from build123d import *

# Parameters (mm, degrees)
SKETCH3_W           = 90
SKETCH3_H           = 50
BOSS_EXTRUDE1_DEPTH = 10
BOSS_EXTRUDE2_DEPTH = 24
SKETCH5_R           = 20
BOSS_EXTRUDE3_DEPTH = 26
SKETCH6_W           = 20
SKETCH6_H           = 27.110350909
CUT_EXTRUDE1_DEPTH  = 15
SKETCH7_W           = 26.369202788
SKETCH7_H           = 10.718734527
CUT_EXTRUDE2_DEPTH  = 35
SKETCH9_W           = 20
SKETCH9_H           = 12
CUT_EXTRUDE3_DEPTH  = 114.798066767


with BuildPart() as part:
    # Sketch3 → Boss-Extrude1 (new body)
    with BuildSketch(Plane.XY):
        Rectangle(SKETCH3_W, SKETCH3_H)
    extrude(amount=BOSS_EXTRUDE1_DEPTH)

    # Sketch4 → Boss-Extrude2 (add)
    with BuildSketch(Plane.XZ.offset(25)):
        Polygon((45, 10), (-45, 10), (-25, 60), (25, 60), align=None)
    extrude(amount=-BOSS_EXTRUDE2_DEPTH)

    # Sketch5 → Boss-Extrude3 (add)
    with BuildSketch(Plane(origin=(0, -1, 0), x_dir=(1, 0, 0), z_dir=(0, 1, 0))):
        with Locations(Location((0, -45, 0), (0, 0, 311.409622109))):
            Circle(SKETCH5_R)
    extrude(amount=BOSS_EXTRUDE3_DEPTH)

    # Sketch6 → Cut-Extrude1 (cut)
    with BuildSketch(Plane(origin=(0, 25, 0), x_dir=(1, 0, 0), z_dir=(0, 1, 0))):
        with Locations((0, -31.444824546)):
            Rectangle(SKETCH6_W, SKETCH6_H)
    extrude(amount=-CUT_EXTRUDE1_DEPTH, mode=Mode.SUBTRACT)

    # Sketch7 → Cut-Extrude2 (cut)
    with BuildSketch(Plane.XZ.offset(25)):
        with Locations((-0.044155161, 65.359367264)):
            Rectangle(SKETCH7_W, SKETCH7_H)
    extrude(amount=-CUT_EXTRUDE2_DEPTH, mode=Mode.SUBTRACT)

    # Sketch9 → Cut-Extrude3 (cut, through all)
    with BuildSketch(Plane(origin=(45, 0, 0), x_dir=(0, 0, -1), z_dir=(1, 0, 0))):
        with Locations((-35, -13)):
            Rectangle(SKETCH9_W, SKETCH9_H)
    extrude(amount=-CUT_EXTRUDE3_DEPTH, mode=Mode.SUBTRACT)


solid = part.part
Read the model definition and answer for the solid it produces. Units are mm, in the model's axes. A direction names the side the tool comes from. Round coordinates to 2 decimals unless told otherwise and drop trailing zeros. Write each loop counter-clockwise with the first axis right and the second up, starting at its lowest first coordinate (ties: lowest second). Pieces come first, ordered by that corner, then holes. Notation, with made-up numbers: (-2.5, 24.5) - (38.5, 24.5) arc R28 ccw to (38.5, 52.5) - close; hole circle Ø4 at (-7, -3.5). An arc over 180 degrees is marked (long way). One line per question, with ' | ' between items. Start each with the question number.
1. Section C-C (z = 31.5) is taken. Determine the outline of the cut face in (x, y), and give its area (3 significant figures).
2. Section A-A (y = -12) is taken. Determine the outline of the cut face in (x, z).
3. Section B-B (x = 30) is taken. Determine the outline of the cut face in (y, z), and give its area (3 significant figures).
4. For a pull along Y with two mould halves and no side action, classify faces 6 (the face through (1, -7, 35)), 7 (the face through (0, -12, 60)), 8 (the face through (0, 10, 35)) as +Y half, -Y half, draft (parallel to the pull), parting line (faces both ways), or undercut.
5. Find the intervals of material crossed by probe 1 along Z at (x, y) = (24, -18); probe 2 along Y at (x, z) = (11.5, 37); probe 3 along Y at (x, z) = (27, 33.5), in increasing order. Write a range as [from, to].
6. Each of these flat-tipped pins is pushed along its axis until it touches: pin 1 (16.5 mm diameter, centred on y = 15.5, z = 36.5, fed in from +X); pin 2 (6 mm diameter, centred on x = 0, z = 39.5, fed in from +Y); pin 3 (1.5 mm diameter, centred on y = 19, z = 54.5, fed in from +X). Where does it stop, or does it pass through?
7. Section D-D (y = 7) is taken. Determine the outline of the cut face in (x, z), and give its area (3 significant figures).
8. For faces 1 (the face through (-1, 12, 10)), 2 (the face through (0, -13, 45)), 3 (the face through (1, -25, 30)), 4 (the face through (-45, 0, 5)), 5 (the face through (0, 18, 45)), determine the directions among +Z, -Z, +X, -X, +Y, -Y from which every point of the face is accessible in a straight line to the end or side of a thin tool.
Filled in:
1) outline: (-36.4, -25) - (36.4, -25) - (36.4, -19) - (-36.4, -19) - close; (-36.4, -7) - (36.4, -7) - (36.4, -1) - (14.76, -1) - (14.76, 25) - (10, 25) - (10, 10) - (-10, 10) - (-10, 25) - (-14.76, 25) - (-14.76, -1) - (-36.4, -1) - close | area: 1,340 mm²
2) outline: (-45, 0) - (45, 0) - (45, 10) - (39, 25) - (-39, 25) - (-45, 10) - close; (-31, 45) - (31, 45) - (25, 60) - (-25, 60) - close
3) outline: (-25, 0) - (25, 0) - (25, 10) - (-1, 10) - (-1, 47.5) - (-25, 47.5) - close; hole (-19, 25) - (-7, 25) - (-7, 45) - (-19, 45) - close | area: 1,160 mm²
4) face 6: undercut | face 7: draft | face 8: +Y half
5) probe 1: [0, 25], [45, 60] | probe 2: [-25, -19], [-7, 25] | probe 3: [-25, -19], [-7, -1]
6) pin 1: x = 20 | pin 2: y = 10 | pin 3: x = 17.98
7) outline: (-45, 0) - (45, 0) - (45, 10) - (-45, 10) - close; (-13.23, 60) arc R20 ccw (long way) to (13.14, 60.08) - (13.14, 60) - close | area: 2,070 mm²
8) face 1: +X, -X, +Y | face 2: +X, -X | face 3: +Z, -Z, +X, -X, -Y | face 4: +Z, -Z, -X, +Y, -Y | face 5: +Y
